Work out the finished part from the listing and answer in its coordinate system (mm). A direction names the side the tool comes from. Coordinates: 2 decimals unless noted, no trailing zeros. Loops run counter-clockwise (first coordinate to the right, second up) from the corner with the lowest first, then second, coordinate; pieces in that order, holes last. Notation, with made-up numbers: (26.25, 77.25) -> (44.25, 77.25) arc R20 cw to (44.25, 92.25) -> close; hole circle Ø3 at (32, 25). An arc over 180 degrees is marked (long way). Use a Markdown table: item, result. Add a question column.
Autodesk Inventor part; units mm, degrees
ref_plane "Start Plane" through (0, 0, -15) normal (0, 0, 1) x (1, 0, 0)
ref_plane "End Plane" through (0, 0, 265) normal (0, 0, 1) x (1, 0, 0)
ref_plane "Work Plane4" through (0, -15, -15) normal (0, 0.7071, -0.7071) x (1, 0, 0)
ref_plane "Start Plane" through (0, 0, -15) normal (0, 0, 1) x (1, 0, 0)
ref_plane "End Plane" through (0, 0, 265) normal (0, 0, 1) x (1, 0, 0)
sketch "Sketch" plane through (0, 0, 0) normal (0, 0, 1) x (1, 0, 0)
  line L0 (-15, -9) -> (-15, 9)
  line L1 (-9, 15) -> (9, 15)
  line L2 (15, 9) -> (15, -9)
  line L3 (9, -15) -> (-9, -15)
  arc A0 (-15, -9) -> (-9, -15) centre (-9, -9) ccw
  arc A1 (-9, 15) -> (-15, 9) centre (-9, 9) ccw
  arc A2 (15, 9) -> (9, 15) centre (9, 9) ccw
  arc A3 (9, -15) -> (15, -9) centre (9, -9) ccw
  arc A4 (-9, 12) -> (-12, 9) centre (-9, 9) ccw
  line L4 (-9, 12) -> (9, 12)
  arc A5 (12, 9) -> (9, 12) centre (9, 9) ccw
  line L5 (12, 9) -> (12, -9)
  arc A6 (9, -12) -> (12, -9) centre (9, -9) ccw
  line L6 (9, -12) -> (-9, -12)
  arc A7 (-12, -9) -> (-9, -12) centre (-9, -9) ccw
  line L7 (-12, -9) -> (-12, 9)
  line L8 (0, 22.7397) -> (0, -22.7397) construction
  line L9 (-22.7397, 0) -> (22.7397, 0) construction
  dimension "d7" = 6
  dimension "d10" = 30
  dimension "d11" = 30
  dimension "d12" = 3
  dimension "d15" = 15
  dimension "d16" = 15
extrude "Body" add sketch "Sketch" along normal up to surface (280 mm away) from surface at -15
sketch "Sketch3" plane through (0, 0, 0) normal (0, 0, 1) x (1, 0, 0)
  line L0 (0, 0) -> (10, 0)
ref_plane "Work Plane3" through (0, 0, 0) normal (0, -1, 0) x (1, 0, 0)
ref_plane "Work Plane4" through (0, -15, -15) normal (0, 0.7071, -0.7071) x (1, 0, 0)
split "Split1" plane through (0, -15, -15) removes the side toward (0, 0.7071, -0.7071)
ref_plane "Work Plane5" through (0, -15, 265) normal (0, 0.7071, 0.7071) x (1, 0, 0)
split "Split2" plane through (0, -15, 265) removes the side toward (0, 0.7071, 0.7071)
sketch "Sketch4" plane through (0, 0, 0) normal (0, -1, 0) x (1, 0, 0)
  line L0 (-2, -15) -> (12, -15)
  line L1 (-2, 265) -> (12, 265)
  dimension "d18" = 280
equation "\"d7\" = G_IR"
equation "\"d10\" = G_H"
equation "\"d11\" = G_W"
equation "\"d12\" = G_T"
equation "\"d15\" = 0.5 * d10"
equation "\"d16\" = 0.5 * d11"
equation "\"d3\" = G_L"
equation "\"G_W\" = 30"
equation "\"G_H\" = 30"
equation "\"G_T\" = 3"
equation "\"G_IR\" = 6"
equation "\"G_L\" = d18"
equation "\"G_OFFSET_START\" = 15"
equation "\"G_OFFSET_END\" = 15"
equation "\"d13\" = -G_OFFSET_START"
equation "\"d14\" = G_OFFSET_END + B_L"
properties part number "DIN EN 10219-2 - 30 x 30 x 3  - 280" material "Steel, Mild"
Item 1: Find the intervals of material crossed by probe 1 along Y at (x, z) = (-8.5, 39); probe 2 along X at (y, z) = (9.5, 62); probe 3 along X at (y, z) = (-11.5, 238), in increasing order.
Item 2: Section B-B (y = 0.25) is taken. Determine the outline of the cut face in (x, z).
Item 3: For faces 1 (the face through (-12, 0, 123)), 2 (the face through (-15, 0, 123)), determine the directions among +Z, -Z, +X, -X, +Y, -Y from which every point of the face is accessible in a straight line to the end or side of a thin tool.
Item 4: Section A-A (x = 6) is taken. Determine the outline of the cut face in (y, z), then the cut area to 3 significant figures.
Item 5: Given pin 1 (5 mm diameter, centred on x = 10.5, y = 11, fed in from +Z); pin 2 (5 mm diameter, centred on y = -12, z = 166.5, fed in from -X); pin 3 (3 mm diameter, centred on x = 11, z = 75, fed in from +Y), each flat-ended and moving along its own axis, determine where each tip first touches the part or whether it passes through.
Item 6: Section C-C (z = 32) is taken. Determine the outline of the cut face in (x, y), then the cut area to 3 significant figures.
Item 7: Section D-D (z = 248) is taken. Determine the outline of the cut face in (x, y), then the cut area to 3 significant figures.
Output:
| question | item | result |
|---|---|---|
| 1 | probe 1 | y = -15 to -12, 12 to 15 |
| 1 | probe 2 | x = -14.98 to -11.96, 11.96 to 14.98 |
| 1 | probe 3 | x = -14.45 to -10.66, 10.66 to 14.45 |
| 2 | outline | (-15, 0.25) -> (-12, 0.25) -> (-12, 249.75) -> (-15, 249.75) -> close; (12, 0.25) -> (15, 0.25) -> (15, 249.75) -> (12, 249.75) -> close |
| 3 | face 1 | +Z, -Z |
| 3 | face 2 | +Z, -Z, -X, +Y, -Y |
| 4 | outline | (-15, -15) -> (-12, -12) -> (-12, 262) -> (-15, 265) -> close; (12, 12) -> (15, 15) -> (15, 235) -> (12, 238) -> close |
| 4 | area | 1,500 mm2 |
| 5 | pin 1 | stops at z = 241 |
| 5 | pin 2 | stops at x = -14.98 |
| 5 | pin 3 | stops at y = 14.98 |
| 6 | outline | (-15, -9) arc R6 ccw to (-9, -15) -> (9, -15) arc R6 ccw to (15, -9) -> (15, 9) arc R6 ccw to (9, 15) -> (-9, 15) arc R6 ccw to (-15, 9) -> close; hole (-12, -9) arc R3 ccw to (-9, -12) -> (9, -12) arc R3 ccw to (12, -9) -> (12, 9) arc R3 ccw to (9, 12) -> (-9, 12) arc R3 ccw to (-12, 9) -> close |
| 6 | area | 301 mm2 |
| 7 | outline | (-15, -9) arc R6 ccw to (-9, -15) -> (9, -15) arc R6 ccw to (15, -9) -> (15, 2) -> (12, 2) -> (12, -9) arc R3 cw to (9, -12) -> (-9, -12) arc R3 cw to (-12, -9) -> (-12, 2) -> (-15, 2) -> close |
| 7 | area | 162 mm2 |
